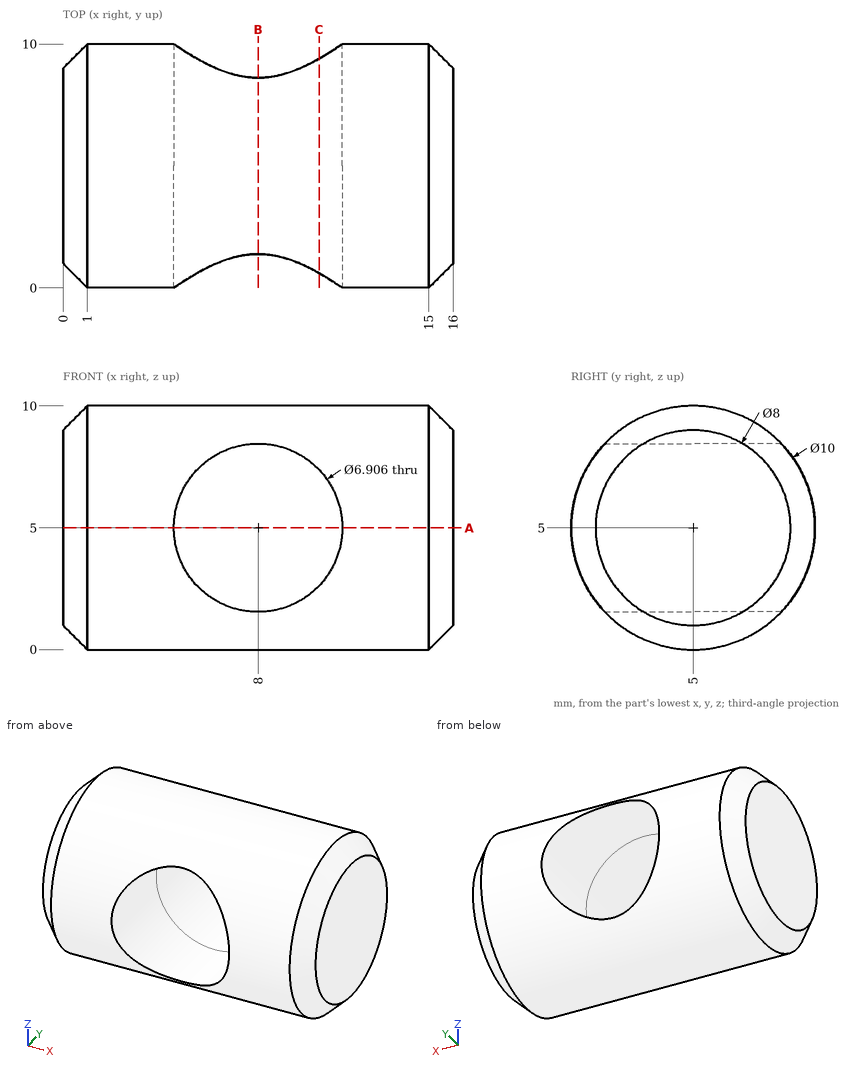
Source: three-view drawing plus pictorial views. Frame: mm from the lowest corner of the part. Give positions to 0.01 mm unless a question says otherwise; leave off trailing zeros. Order: outer loops, then holes, each group sorted by start corner. A loop starts at its lowest first (then second) coordinate and runs counter-clockwise, first axis right, second up.
1. Section C-C on x = 10.5. Return the cut outline in (y, z).
Derived:
outline: (0.6, 2.62) arc R5 ccw to (9.4, 2.62) - close; (0.6, 7.38) - (9.4, 7.38) arc R5 ccw to start
2. Material intervals for L1, parallel to X at y = 8.5, z = 2; L2, parallel to Z at x = 8.75, y = 2; L3, parallel to Z at x = 8, y = 7.75 (1 decimal), sorted ascending.
Derived:
L1: x = 0.61 to 6.29, 9.71 to 15.39
L2: z = 1 to 1.63, 8.37 to 9
L3: z = 0.8 to 1.5, 8.5 to 9.2
3. Section B-B on x = 8. Return the cut outline in (y, z).
Derived:
outline: (1.38, 1.55) arc R5 ccw to (8.62, 1.55) - close; (1.38, 8.45) - (8.62, 8.45) arc R5 ccw to start
4. Pin query (flat end, axial travel): pin 1 (6 mm diameter, centred on x = 9, y = 1.5, fed in from -Z) (1 decimal); pin 2 (1 mm diameter, centred on x = 13, z = 6.5, fed in from +Y); pin 3 (1 mm diameter, centred on y = 8.5, z = 2, fed in from -X). Return the tip coordinate at first contact, or that it passes through.
Derived:
pin 1: stops at z = 0
pin 2: stops at y = 9.9
pin 3: stops at x = 0.11
5. Section A-A on z = 5. Return the cut outline in (x, y).
Derived:
outline: (0, 1) - (1, 0) - (4.55, 0) - (4.55, 10) - (1, 10) - (0, 9) - close; (11.45, 0) - (15, 0) - (16, 1) - (16, 9) - (15, 10) - (11.45, 10) - close
